Source: three-view drawing plus pictorial views. Frame: mm from the lowest corner of the part. A direction names the side the tool comes from. Round coordinates to 2 decimals unless told otherwise and drop trailing zeros. Write each loop counter-clockwise with the first axis right and the second up, starting at its lowest first coordinate (ties: lowest second). Pieces come first, ordered by that corner, then holes.
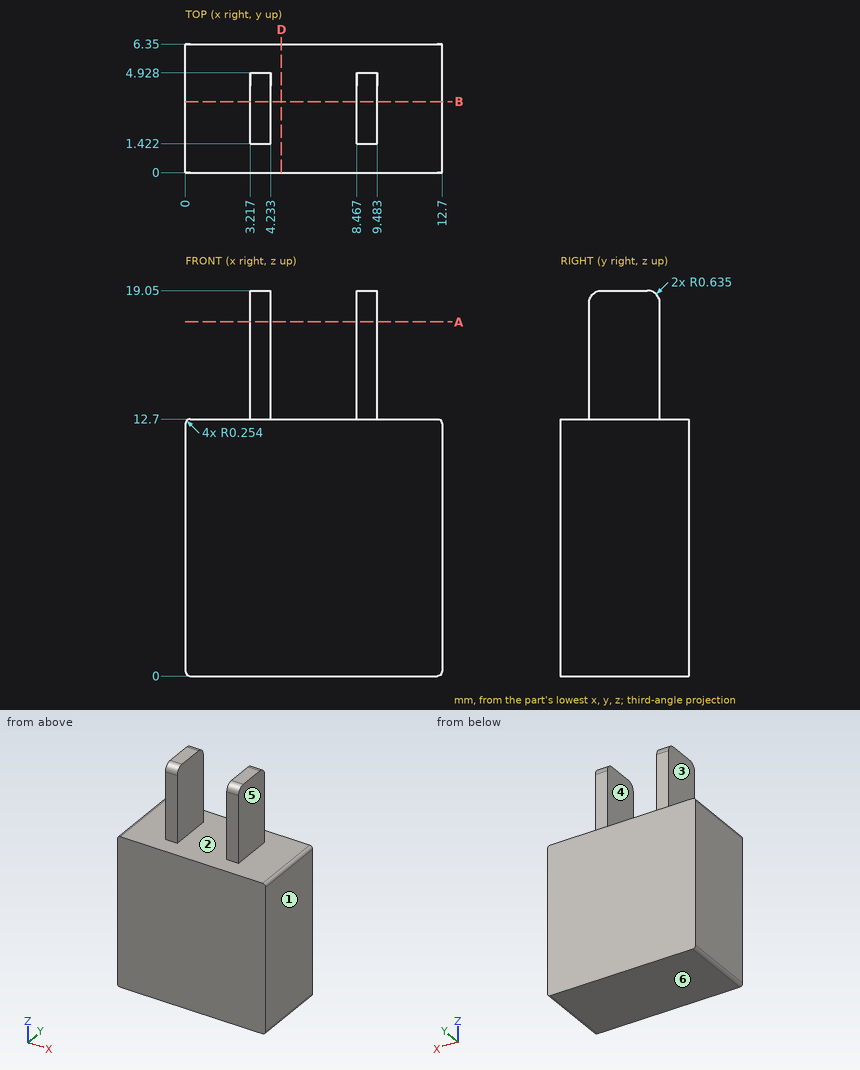
1) Line query: probe 1 along X at (y, z) = (3.75, 17); probe 2 along Z at (x, y) = (8, 4); probe 3 along Y at (x, z) = (9, 15.25). Output: solid intervals per line, ascending.
2) Section A-A on z = 17.5. Output: boundary loops of the cut face in (x, y).
3) Section B-B on y = 3.5. Output: boundary loops of the cut face in (x, z), plus the area to 3 significant figures.
4) Reachability of the marked faces 4, 5 and 6 from +Z, -Z, +X, -X, +Y, -Y: full face, straight path, thin tool, end or side. Return the list, or none.
5) First-contact query: P1, Ø1.1, axis at y = 4, z = 16.5, coming from the -X side; P2, Ø1.5, axis at x = 4.5, y = 1, coming from the -Z side; P3, Ø1, axis at x = 1.5, z = 15.5, coming from the -Y side; P4, Ø1.1, axis at y = 3.5, z = 15, coming from the +X side. Flat tips, straight axial feed; report the tip coordinate or a pass-through.
6) Draft query along X for the marked faces 1, 2 and 3. Return one class per face: pulls with the +X half, pulls with the -X half, needs draft (parallel to the pull), parting line crosses it, or undercut.
7) Section D-D on x = 4.75. Output: boundary loops of the cut face in (y, z).
Filled in:
1. probe 1: x = 3.22 to 4.23, 8.47 to 9.48
1. probe 2: z = 0 to 12.7
1. probe 3: y = 1.42 to 4.93
2. outline: (3.22, 1.42) - (4.23, 1.42) - (4.23, 4.93) - (3.22, 4.93) - close; (8.47, 1.42) - (9.48, 1.42) - (9.48, 4.93) - (8.47, 4.93) - close
3. outline: (0, 0.25) arc R0.25 ccw to (0.25, 0) - (12.45, 0) arc R0.25 ccw to (12.7, 0.25) - (12.7, 12.45) arc R0.25 ccw to (12.45, 12.7) - (9.48, 12.7) - (9.48, 19.05) - (8.47, 19.05) - (8.47, 12.7) - (4.23, 12.7) - (4.23, 19.05) - (3.22, 19.05) - (3.22, 12.7) - (0.25, 12.7) arc R0.25 ccw to (0, 12.45) - close
3. area: 174 mm2
4. face 4: +Z, +Y, -Y
4. face 5: +Z, +X, +Y, -Y
4. face 6: -Z, +X, -X, +Y, -Y
5. P1: stops at x = 3.22
5. P2: stops at z = 0
5. P3: passes through
5. P4: stops at x = 9.48
6. face 1: pulls with the +X half
6. face 2: undercut
6. face 3: pulls with the -X half
7. outline: (0, 0) - (6.35, 0) - (6.35, 12.7) - (0, 12.7) - close
